Could you check a few things on this model? Use its own coordinates, in mm. A direction names the side the tool comes from. Coordinates: 2 decimals unless noted, no trailing zeros. Order: outer loops, then holes, each group sorted by start corner. A loop starts at its lowest first (then second) coordinate and runs counter-clockwise, first axis right, second up. Notation, with made-up numbers: (-2, 45) -> (34, 45) arc R13 cw to (34, 51) -> close; hole circle Ø11 at (4.5, 24.25). An arc over 180 degrees is marked (long way). Use a Markdown table: item, result. Add a question column.
1) If we section it at C-C (y = 2.1): Give the number of separate pieces and of enclosed holes in the cut face, plus the area to 3 significant figures.
2) Thinking about a two-plate mould opening in X: for faces 1 (the flat face through (75, 2, -3)), 2 (the flat face through (35, 2, -3)), 3 (the flat face through (20, 2, -1)), 4 (the flat face through (1, 2, -40)), which applies, +X half, -X half, draft (parallel to the pull), parting line (faces both ways), or undercut?
3) If I drill on L1, parallel to X at y = 0.95, z = -41.7; L2, parallel to Z at x = 134, y = 1.75; L3, parallel to X at y = 2.2, z = -28, over which ranges is the centre line in solid material (lowest first)? Write a range as [from, to].
4) Which directions (+Z, -Z, +X, -X, +Y, -Y) give clear straight access to the entire face, cutting with the end or side of a thin tool? Please do faces 5 (the flat face through (110, 2, -1)), 6 (the flat face through (138, 2, -3)), 7 (the flat face through (1, 2, -20)), 8 (the flat face through (12, 2, -3)).
5) If we section it at A-A (z = -41.7): Write out the boundary of the cut face in (x, y).
6) If we section it at B-B (x = 75): Write out the boundary of the cut face in (y, z).
7) Will these pins go through, and if not, where does the flat tip stop? pin 1 Ø0.9 at (y, z) = (1, -1.5) entering from -X; pin 2 Ø1.5 at (x, y) = (54, 1) entering from +Z; pin 3 Ø0.9 at (x, y) = (1.5, 1.5) entering from -Z; pin 4 Ø2.5 at (x, z) = (75, -41.7) entering from +Y.
8) If we section it at D-D (x = 9): Write out the boundary of the cut face in (y, z).
```python
from build123d import *

# Parameters (mm, degrees)
MDFESB_W       = 150
MDFESB_H       = 50
MDF_DEPTH      = 3
ENCAIXEESB_W   = 10
ENCAIXEESB_H   = 3
ENCAIXEESB_W_2 = 3
ENCAIXEESB_H_2 = 10
ENCAIXE_DEPTH  = 3
USESB_R        = 2.1
US_DEPTH       = 3


with BuildPart() as part:
    # mdfEsb → mdf (new body)
    with BuildSketch(Plane(origin=(0, 0, 0), x_dir=(1, 0, 0), z_dir=(0, 1, 0))):
        with Locations((75, 25)):
            Rectangle(MDFESB_W, MDFESB_H)
    extrude(amount=MDF_DEPTH)

    # encaixeEsb → encaixe (cut)
    with BuildSketch(Plane(origin=(0, 3, 0), x_dir=(1, 0, 0), z_dir=(0, 1, 0))):
        Polygon((0, 0), (20, 0), (20, 3), (3, 3), (3, 10), (0, 10), (0, 3), align=None)
        Polygon((150, 0), (130, 0), (130, 3), (147, 3), (147, 10), (150, 10), (150, 3), align=None)
        with Locations((35, 1.5)):
            Rectangle(ENCAIXEESB_W, ENCAIXEESB_H)
        with Locations((55, 1.5)):
            Rectangle(ENCAIXEESB_W, ENCAIXEESB_H)
        with Locations((75, 1.5)):
            Rectangle(ENCAIXEESB_W, ENCAIXEESB_H)
        with Locations((95, 1.5)):
            Rectangle(ENCAIXEESB_W, ENCAIXEESB_H)
        with Locations((115, 1.5)):
            Rectangle(ENCAIXEESB_W, ENCAIXEESB_H)
        with Locations((1.5, 25)):
            Rectangle(ENCAIXEESB_W_2, ENCAIXEESB_H_2)
        with Locations((1.5, 45)):
            Rectangle(ENCAIXEESB_W_2, ENCAIXEESB_H_2)
        with Locations((1.5, 65)):
            Rectangle(ENCAIXEESB_W_2, ENCAIXEESB_H_2)
        with Locations((1.5, 85)):
            Rectangle(ENCAIXEESB_W_2, ENCAIXEESB_H_2)
        with Locations((1.5, 105)):
            Rectangle(ENCAIXEESB_W_2, ENCAIXEESB_H_2)
        with Locations((148.5, 105)):
            Rectangle(ENCAIXEESB_W_2, ENCAIXEESB_H_2)
        with Locations((148.5, 85)):
            Rectangle(ENCAIXEESB_W_2, ENCAIXEESB_H_2)
        with Locations((148.5, 65)):
            Rectangle(ENCAIXEESB_W_2, ENCAIXEESB_H_2)
        with Locations((148.5, 45)):
            Rectangle(ENCAIXEESB_W_2, ENCAIXEESB_H_2)
        with Locations((148.5, 25)):
            Rectangle(ENCAIXEESB_W_2, ENCAIXEESB_H_2)
    extrude(amount=-ENCAIXE_DEPTH, mode=Mode.SUBTRACT)

    # USEsb → US (cut)
    with BuildSketch(Plane(origin=(0, 3, 0), x_dir=(1, 0, 0), z_dir=(0, 1, 0))):
        with Locations(Location((75, 41.7, 0), (0, 0, 270))):
            Circle(USESB_R)
        with Locations(Location((75, 10, 0), (0, 0, 270))):
            Circle(USESB_R)
    extrude(amount=-US_DEPTH, mode=Mode.SUBTRACT)


solid = part.part
```
Answer sheet:
| question | item | result |
|---|---|---|
| 1 | separate pieces | 1 |
| 1 | enclosed holes | 2 |
| 1 | area | 7,040 mm2 |
| 2 | face 1 | undercut |
| 2 | face 2 | undercut |
| 2 | face 3 | -X half |
| 2 | face 4 | draft |
| 3 | L1 | [3, 72.9], [77.1, 147] |
| 3 | L2 | [-50, -3] |
| 3 | L3 | [3, 147] |
| 4 | face 5 | +Z, +Y, -Y |
| 4 | face 6 | +Z, +X, +Y, -Y |
| 4 | face 7 | -X, +Y, -Y |
| 4 | face 8 | +Z, -X, +Y, -Y |
| 5 | outline | (3, 0) -> (72.9, 0) -> (72.9, 3) -> (3, 3) -> close; (77.1, 0) -> (147, 0) -> (147, 3) -> (77.1, 3) -> close |
| 6 | outline | (0, -50) -> (3, -50) -> (3, -43.8) -> (0, -43.8) -> close; (0, -39.6) -> (3, -39.6) -> (3, -12.1) -> (0, -12.1) -> close; (0, -7.9) -> (3, -7.9) -> (3, -3) -> (0, -3) -> close |
| 7 | pin 1 | x = 20 |
| 7 | pin 2 | z = -3 |
| 7 | pin 3 | z = -40 |
| 7 | pin 4 | through |
| 8 | outline | (0, -50) -> (3, -50) -> (3, -3) -> (0, -3) -> close |
